```python
from build123d import *

# Parameters (mm, degrees)
F0_R     = 8.5
F1_DEPTH = 4
F2_R     = 5.5
F3_DEPTH = 100
F4_R     = 1
F5_DEPTH = 114.9
F6_R     = 1.5
F7_DEPTH = 80


with BuildPart() as f1:
    # F0 (on Top) → F1 (new body)
    with BuildSketch(Plane.XY):
        Circle(F0_R)
    extrude(amount=F1_DEPTH)

    # F2 (on Top) → F3 (join)
    with BuildSketch(Plane.XY):
        Circle(F2_R)
    extrude(amount=F3_DEPTH)

    # F4 (on face) → F5 (cut)
    with BuildSketch(Plane.XY.offset(100)):
        Circle(F4_R)
    extrude(amount=-F5_DEPTH, mode=Mode.SUBTRACT)

    # F6 (on Top) → F7 (cut)
    with BuildSketch(Plane.XY):
        Circle(F6_R)
    extrude(amount=F7_DEPTH, mode=Mode.SUBTRACT)


solid = f1.part
```
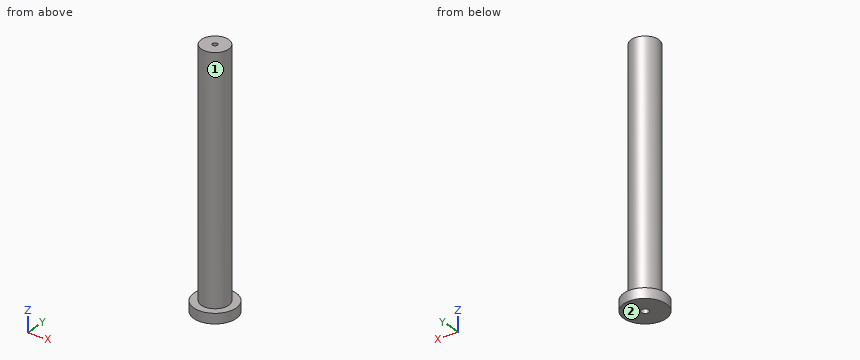
Input: part model. Units: mm. Frame: model coordinates. Face numbers are marked on the shaded views. A direction names the side the tool comes from. Coordinates: 2 decimals unless noted, no trailing zeros. Loops run counter-clockwise (first coordinate to the right, second up) from the corner with the lowest first, then second, coordinate; pieces in that order, holes last.
Q1. Section C-C, the plane z = 81.5. Return the cut outline in (x, y).
Results are:
outline: circle Ø11 at (0, 0); hole circle Ø2 at (0, 0)
Q2. Line query: line 1 along Y through (x, z) = (0, 58.5); line 2 along Z through (x, y) = (-4.5, 7); line 3 along Y through (x, z) = (0.5, 15.5). Output: solid intervals per line, ascending.
Results are:
line 1: y = -5.5 to -1.5, 1.5 to 5.5
line 2: z = 0 to 4
line 3: y = -5.48 to -1.41, 1.41 to 5.48
Q3. Set-up query: the marked faces 1 and 2. Return all of +Z, -Z, +X, -X, +Y, -Y with unobstructed straight access to the full face (end or side cutting, diameter ignored); none if empty.
Results are:
face 1: +Z
face 2: -Z, +X, -X, +Y, -Y
Q4. Section D-D, the plane x = 4.5. Return the cut outline in (y, z), and give its area (3 significant figures).
Results are:
outline: (-7.21, 0) - (7.21, 0) - (7.21, 4) - (3.16, 4) - (3.16, 100) - (-3.16, 100) - (-3.16, 4) - (-7.21, 4) - close
area: 665 mm2
Q5. Contact query for flat-ended pins moving along their axis: pin 1 (1.5 mm diameter, centred on x = 1.5, z = 38.5, fed in from +Y); pin 2 (1.8 mm diameter, centred on x = 0, y = 0, fed in from +Z); pin 3 (2 mm diameter, centred on x = -4, z = 23, fed in from +Y); pin 4 (8 mm diameter, centred on y = -5, z = 26.5, fed in from -X). Output: stop coordinate, or through.
Results are:
pin 1: stops at y = 5.45
pin 2: passes through
pin 3: stops at y = 4.61
pin 4: stops at x = -5.41
Q6. Section A-A, the plane y = 0. Return the cut outline in (x, z), and give its area (3 significant figures).
Results are:
outline: (-8.5, 0) - (-1.5, 0) - (-1.5, 80) - (-1, 80) - (-1, 100) - (-5.5, 100) - (-5.5, 4) - (-8.5, 4) - close; (1, 80) - (1.5, 80) - (1.5, 0) - (8.5, 0) - (8.5, 4) - (5.5, 4) - (5.5, 100) - (1, 100) - close
area: 844 mm2
